Geometry: final body of the model. Coordinates: model frame, mm. Face numbers are marked on the shaded views. Give positions to 0.01 mm unless a question says otherwise; leave off trailing zeros. Order: outer loops, then holes, each group sorted by start corner. A loop starts at its lowest first (then second) coordinate and runs counter-clockwise, first axis right, second up. Notation, with made-up numbers: (5.25, -22) - (15.25, -22) arc R35 cw to (15.25, 13) - close; hole circle Ø10 at (52.25, 67.25). An arc over 180 degrees is marked (long way). One line per item, written item: value.
```python
from build123d import *

# Parameters (mm, degrees)
F0_W      = 110
F0_H      = 110
F1_DEPTH  = 30
F2_R      = 25
F2_R_2    = 17.5
F3_DEPTH  = 10
F3_FACE_R = 17.5
F4_DEPTH  = 30.001
F5_W      = 10
F5_H      = 19
F6_DEPTH  = 110.001
F7_R      = 4
F8_DEPTH  = 25.4


with BuildPart() as f1:
    # F0 (on Front) → F1 (new body)
    with BuildSketch(Plane.XZ):
        Rectangle(F0_W, F0_H)
    extrude(amount=F1_DEPTH)

    # F2 (on face) → F3 (cut)
    with BuildSketch(Plane.XZ.offset(30)):
        Circle(F2_R)
        Circle(F2_R_2, mode=Mode.SUBTRACT)
    extrude(amount=-F3_DEPTH, mode=Mode.SUBTRACT)

    # F3_face (on face) → F4 (cut, through all)
    with BuildSketch(Plane.XZ.offset(30)):
        Circle(F3_FACE_R)
    extrude(amount=-F4_DEPTH, mode=Mode.SUBTRACT)

    # F5 (on face) → F6 (cut, through all)
    with BuildSketch(Plane.XY.offset(55)):
        with Locations((-55, -15)):
            Rectangle(F5_W, F5_H)
        with Locations((55, -15)):
            Rectangle(F5_W, F5_H)
    extrude(amount=-F6_DEPTH, mode=Mode.SUBTRACT)

    # F7 (on face) → F8 (cut)
    with BuildSketch(Plane.XY.offset(55)):
        with Locations((0, -15)):
            Circle(F7_R)
    extrude(amount=-F8_DEPTH, mode=Mode.SUBTRACT)


solid = f1.part
```
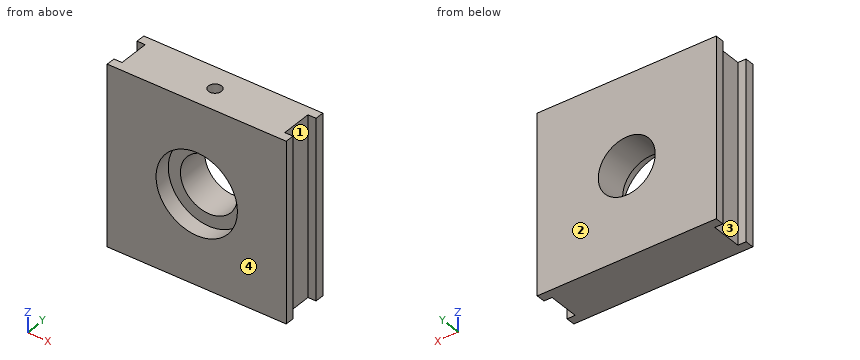
1) Section B-B, the plane x = 0. Return loops of the section in (y, z), then the cut area to 3 significant figures.
Answers below:
outline: (-30, -55) - (0, -55) - (0, -17.5) - (-20, -17.5) - (-20, -25) - (-30, -25) - close; (-30, 25) - (-20, 25) - (-20, 17.5) - (0, 17.5) - (0, 55) - (-11, 55) - (-11, 29.6) - (-19, 29.6) - (-19, 55) - (-30, 55) - close
area: 1,900 mm^2
2) Section D-D, the plane x = -20. Return loops of the section in (y, z), then the cut area to 3 significant figures.
Answers below:
outline: (-30, -55) - (0, -55) - (0, 55) - (-30, 55) - (-30, 15) - (-20, 15) - (-20, -15) - (-30, -15) - close
area: 3,000 mm^2
3) Section C-C, the plane y = -9.5. Return loops of the section in (x, z).
Answers below:
outline: (-50, -55) - (50, -55) - (50, 55) - (-50, 55) - close; hole circle Ø35 at (0, 0)
4) First-contact query: pin 1 (2.5 mm diameter, centred on x = -0.5, y = -15.5, fed in from +Z); pin 2 (5 mm diameter, centred on y = -16, z = 3.5, fed in from -X). Flat tips, straight axial feed; report the tip coordinate or a pass-through.
Answers below:
pin 1: z = 29.6
pin 2: x = -50
5) Mould query, pull axis Y, two halves, no side actions, for the marked faces 1, 2, 3 and 4. Classes: released by +Y, released by -Y, zero draft, split by the parting line, or undercut.
Answers below:
face 1: undercut
face 2: released by +Y
face 3: undercut
face 4: released by -Y
6) Material intervals for line 1 along Z through (x, y) = (0, -6); line 2 along Z through (x, y) = (0, -15.5); line 3 along Y through (x, z) = (0, 41.25), sorted ascending.
Answers below:
line 1: -55 to -17.5, 17.5 to 55
line 2: -55 to -17.5, 17.5 to 29.6
line 3: -30 to -19, -11 to 0
7) Section A-A, the plane z = 0. Return loops of the section in (x, y).
Answers below:
outline: (-55, -30) - (-25, -30) - (-25, -20) - (-17.5, -20) - (-17.5, 0) - (-55, 0) - (-55, -5.5) - (-50, -5.5) - (-50, -24.5) - (-55, -24.5) - close; (17.5, -20) - (25, -20) - (25, -30) - (55, -30) - (55, -24.5) - (50, -24.5) - (50, -5.5) - (55, -5.5) - (55, 0) - (17.5, 0) - close
